from build123d import *

# Parameters (mm, degrees)
SKETCH1_R           = 3.4
BOSS_EXTRUDE2_DEPTH = 100
FILLET5_R           = 2.5
FILLET6_R           = 1.5
FILLET7_R           = 1.5
FILLET8_R           = 1
SKETCH3_R           = 3.4
BOSS_EXTRUDE3_DEPTH = 140


with BuildPart() as part:
    # Sketch1 → Boss-Extrude2 (new body)
    with BuildSketch(Plane(origin=(0, 0, 0), x_dir=(0, 0, -1), z_dir=(1, 0, 0))):
        Polygon((10.9, 0), (10.9, 2.4), (6.75, 2.4), (6.75, 5.05), (10.9, 9.2), (19.1, 9.2), (23.25, 5.05), (23.25, 2.4), (19.1, 2.4), (19.1, 0), (30, 0), (30, 10.9), (27.6, 10.9), (27.6, 6.75), (24.95, 6.75), (20.8, 10.9), (20.8, 19.1), (24.95, 23.25), (27.6, 23.25), (27.6, 19.1), (30, 19.1), (30, 30), (19.1, 30), (19.1, 27.6), (23.25, 27.6), (23.25, 24.95), (19.1, 20.8), (10.9, 20.8), (6.75, 24.95), (6.75, 27.6), (10.9, 27.6), (10.9, 30), (0, 30), (0, 19.1), (2.4, 19.1), (2.4, 23.25), (5.05, 23.25), (9.2, 19.1), (9.2, 10.9), (5.05, 6.75), (2.4, 6.75), (2.4, 10.9), (0, 10.9), (0, 0), align=None)
        with Locations((15, 15)):
            Circle(SKETCH1_R, mode=Mode.SUBTRACT)
    extrude(amount=BOSS_EXTRUDE2_DEPTH)

    # Fillet5
    fillet5_edges = [part.edges().sort_by_distance(p)[0] for p in [
        (50, 30, 0),
        (50, 30, -30),
        (50, 0, -30),
        (50, 0, 0),
    ]]
    fillet(fillet5_edges, radius=FILLET5_R)

    # Fillet6
    fillet6_edges = [part.edges().sort_by_distance(p)[0] for p in [
        (50, 10.9, -9.2),
        (50, 19.1, -9.2),
        (50, 19.1, -20.8),
        (50, 10.9, -20.8),
        (50, 9.2, -19.1),
        (50, 9.2, -10.9),
    ]]
    fillet(fillet6_edges, radius=FILLET6_R)

    # Fillet7
    fillet7_edges = [part.edges().sort_by_distance(p)[0] for p in [
        (50, 20.8, -10.9),
        (50, 20.8, -19.1),
    ]]
    fillet(fillet7_edges, radius=FILLET7_R)

    # Fillet8
    fillet8_edges = [part.edges().sort_by_distance(p)[0] for p in [
        (50, 6.75, -2.4),
        (50, 23.25, -2.4),
        (50, 27.6, -6.75),
        (50, 27.6, -23.25),
        (50, 23.25, -27.6),
        (50, 6.75, -27.6),
        (50, 2.4, -23.25),
        (50, 2.4, -6.75),
    ]]
    fillet(fillet8_edges, radius=FILLET8_R)

    # Sketch3 → Boss-Extrude3 (add)
    with BuildSketch(Plane(origin=(0, 0, 0), x_dir=(0, 0, -1), z_dir=(1, 0, 0))):
        with BuildLine():
            Line((10.9, 27.6), (10.9, 30))
            Line((10.9, 30), (2.5, 30))
            ThreePointArc((2.5, 30), (0.732233047, 29.267766953), (0, 27.5))
            Line((0, 27.5), (0, 19.1))
            Line((0, 19.1), (2.4, 19.1))
            Line((2.4, 19.1), (2.4, 22.25))
            ThreePointArc((2.4, 22.25), (2.692893219, 22.957106781), (3.4, 23.25))
            Line((3.4, 23.25), (5.05, 23.25))
            Line((5.05, 23.25), (8.760660172, 19.539339828))
            ThreePointArc((8.760660172, 19.539339828), (9.085819299, 19.052704805), (9.2, 18.478679656))
            Line((9.2, 18.478679656), (9.2, 11.521320344))
            ThreePointArc((9.2, 11.521320344), (9.085819299, 10.947295195), (8.760660172, 10.460660172))
            Line((8.760660172, 10.460660172), (5.05, 6.75))
            Line((5.05, 6.75), (3.4, 6.75))
            ThreePointArc((3.4, 6.75), (2.692893219, 7.042893219), (2.4, 7.75))
            Line((2.4, 7.75), (2.4, 10.9))
            Line((2.4, 10.9), (0, 10.9))
            Line((0, 10.9), (0, 2.5))
            ThreePointArc((0, 2.5), (0.732233047, 0.732233047), (2.5, 0))
            Line((2.5, 0), (10.9, 0))
            Line((10.9, 0), (10.9, 2.4))
            Line((10.9, 2.4), (7.75, 2.4))
            ThreePointArc((7.75, 2.4), (7.042893219, 2.692893219), (6.75, 3.4))
            Line((6.75, 3.4), (6.75, 5.05))
            Line((6.75, 5.05), (10.460660172, 8.760660172))
            ThreePointArc((10.460660172, 8.760660172), (10.947295195, 9.085819299), (11.521320344, 9.2))
            Line((11.521320344, 9.2), (18.478679656, 9.2))
            ThreePointArc((18.478679656, 9.2), (19.052704805, 9.085819299), (19.539339828, 8.760660172))
            Line((19.539339828, 8.760660172), (23.25, 5.05))
            Line((23.25, 5.05), (23.25, 3.4))
            ThreePointArc((23.25, 3.4), (22.957106781, 2.692893219), (22.25, 2.4))
            Line((22.25, 2.4), (19.1, 2.4))
            Line((19.1, 2.4), (19.1, 0))
            Line((19.1, 0), (27.5, 0))
            ThreePointArc((27.5, 0), (29.267766953, 0.732233047), (30, 2.5))
            Line((30, 2.5), (30, 10.9))
            Line((30, 10.9), (27.6, 10.9))
            Line((27.6, 10.9), (27.6, 7.75))
            ThreePointArc((27.6, 7.75), (27.307106781, 7.042893219), (26.6, 6.75))
            Line((26.6, 6.75), (24.95, 6.75))
            Line((24.95, 6.75), (21.239339828, 10.460660172))
            ThreePointArc((21.239339828, 10.460660172), (20.914180701, 10.947295195), (20.8, 11.521320344))
            Line((20.8, 11.521320344), (20.8, 18.478679656))
            ThreePointArc((20.8, 18.478679656), (20.914180701, 19.052704805), (21.239339828, 19.539339828))
            Line((21.239339828, 19.539339828), (24.95, 23.25))
            Line((24.95, 23.25), (26.6, 23.25))
            ThreePointArc((26.6, 23.25), (27.307106781, 22.957106781), (27.6, 22.25))
            Line((27.6, 22.25), (27.6, 19.1))
            Line((27.6, 19.1), (30, 19.1))
            Line((30, 19.1), (30, 27.5))
            ThreePointArc((30, 27.5), (29.267766953, 29.267766953), (27.5, 30))
            Line((27.5, 30), (19.1, 30))
            Line((19.1, 30), (19.1, 27.6))
            Line((19.1, 27.6), (22.25, 27.6))
            ThreePointArc((22.25, 27.6), (22.957106781, 27.307106781), (23.25, 26.6))
            Line((23.25, 26.6), (23.25, 24.95))
            Line((23.25, 24.95), (19.539339828, 21.239339828))
            ThreePointArc((19.539339828, 21.239339828), (19.052704805, 20.914180701), (18.478679656, 20.8))
            Line((18.478679656, 20.8), (11.521320344, 20.8))
            ThreePointArc((11.521320344, 20.8), (10.947295195, 20.914180701), (10.460660172, 21.239339828))
            Line((10.460660172, 21.239339828), (6.75, 24.95))
            Line((6.75, 24.95), (6.75, 26.6))
            ThreePointArc((6.75, 26.6), (7.042893219, 27.307106781), (7.75, 27.6))
            Line((7.75, 27.6), (10.9, 27.6))
        make_face()
        with Locations((15, 15)):
            Circle(SKETCH3_R, mode=Mode.SUBTRACT)
    extrude(amount=-BOSS_EXTRUDE3_DEPTH)


solid = part.part
The listing builds one solid part. Answer for the finished solid, in the listing's coordinates (mm). A direction names the side the tool comes from. Give positions to 0.01 mm unless a question says otherwise; leave off trailing zeros. Write each loop counter-clockwise with the first axis right and the second up, starting at its lowest first coordinate (ties: lowest second). Pieces come first, ordered by that corner, then holes.
Item 1: Find the intervals of material crossed by line 1 along Y through (x, z) = (-5, -14.75); line 2 along Y through (x, z) = (42.5, -7); line 3 along Y through (x, z) = (34.5, -22.25), in increasing order.
Item 2: Which of the six approach directions +Z, -Z, +X, -X, +Y, -Y give full straight-line access (tool end or side, diameter ignored) to faces 1 (the flat face through (-18, 20.8, -15)), 2 (the flat face through (-18, 15, -20.8)), 3 (the flat face through (-18, 9.2, -15)), 4 (the flat face through (-18.3, 8.6, -6.9))?
Item 3: Determine the mould class of faces 5 (the flat face through (-18, 15, -9.2)), 6 (the flat face through (-18, 0, -7)), 7 (the flat face through (-18.3, 23.1, -21.4)), 8 (the flat face through (-18, 30, -23)) for opening direction Y: released by +Y, released by -Y, zero draft, split by the parting line, or undercut.
Item 4: Section A-A, the plane z = -15 is taken. Write down the section's boundary in (x, y).
Item 5: Section B-B, the plane y = 15 is taken. Write down the section's boundary in (x, z).
Item 6: Flat-ended cylindrical pins translate along their axes: P1, Ø5, axis at x = 70.5, y = 15.5, coming from the +Z side; P2, Ø2.5, axis at x = -21, z = -1, coming from the -Y side; P3, Ø0.7, axis at x = -1, z = -29, coming from the +Y side. Find the tip coordinate at first contact, or state that the pin passes through.
Completed:
1. line 1: y = 9.2 to 11.61, 18.39 to 20.8
1. line 2: y = 0 to 2.74, 5.3 to 8.7, 21.3 to 24.7, 27.26 to 30
1. line 3: y = 0 to 2.4, 6.05 to 9.45, 20.55 to 23.95, 27.6 to 30
2. face 1: +X, -X, +Y
2. face 2: -Z, +X, -X
2. face 3: +X, -X, -Y
2. face 4: +X, -X
3. face 5: undercut
3. face 6: released by -Y
3. face 7: undercut
3. face 8: released by +Y
4. outline: (-140, 9.2) - (100, 9.2) - (100, 11.6) - (-140, 11.6) - close; (-140, 18.4) - (100, 18.4) - (100, 20.8) - (-140, 20.8) - close
5. outline: (-140, -20.8) - (100, -20.8) - (100, -18.4) - (-140, -18.4) - close; (-140, -11.6) - (100, -11.6) - (100, -9.2) - (-140, -9.2) - close
6. P1: stops at z = -9.2
6. P2: stops at y = 0.01
6. P3: stops at y = 29.72
